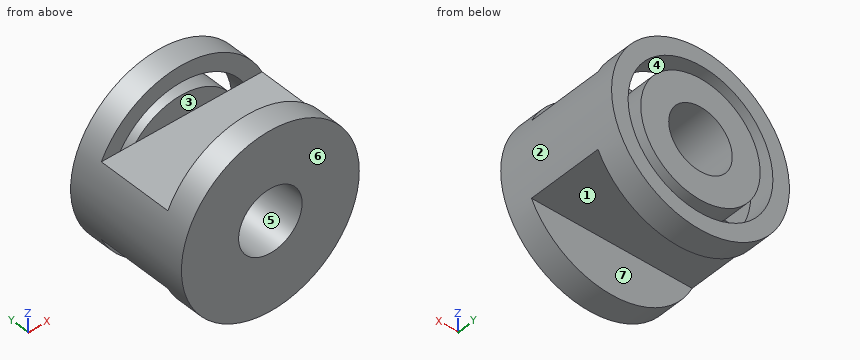
from build123d import *

# Parameters (mm, degrees)
ESQUISSE1_R                  = 3.5
BOSS_EXTRU_1_DEPTH           = 5
ESQUISSE2_R                  = 2.85
ESQUISSE2_R_2                = 2.35
ENL_V_MAT_EXTRU_1_DEPTH      = 1
ESQUISSE3_R                  = 1.25
ENL_V_MAT_EXTRU_2_DEPTH      = 6
ESQUISSE4_W                  = 2
ESQUISSE4_H                  = 3
ENL_V_MAT_EXTRU_3_DEPTH      = 4.5
ENL_V_MAT_EXTRU_3_DEPTH_BACK = 4.5


with BuildPart() as part:
    # Esquisse1 → Boss.-Extru.1 (new body)
    with BuildSketch(Plane(origin=(0, 0, 0), x_dir=(1, 0, 0), z_dir=(0, 1, 0))):
        Circle(ESQUISSE1_R)
    extrude(amount=BOSS_EXTRU_1_DEPTH)

    # Esquisse2 → Enlèv. mat.-Extru.1 (cut)
    with BuildSketch(Plane(origin=(0, 5, 0), x_dir=(1, 0, 0), z_dir=(0, 1, 0))):
        Circle(ESQUISSE2_R)
        Circle(ESQUISSE2_R_2, mode=Mode.SUBTRACT)
    extrude(amount=-ENL_V_MAT_EXTRU_1_DEPTH, mode=Mode.SUBTRACT)

    # Esquisse3 → Enlèv. mat.-Extru.2 (cut, through all)
    with BuildSketch(Plane(origin=(0, 5, 0), x_dir=(1, 0, 0), z_dir=(0, 1, 0))):
        Circle(ESQUISSE3_R)
    extrude(amount=-ENL_V_MAT_EXTRU_2_DEPTH, mode=Mode.SUBTRACT)

    # Esquisse4 → Enlèv. mat.-Extru.3 (cut, two sides)
    with BuildSketch(Plane(origin=(0, 0, 0), x_dir=(0, 0, -1), z_dir=(1, 0, 0))) as enl_v_mat_extru_3_sk:
        with Locations((-2.5, 2.5)):
            Rectangle(ESQUISSE4_W, ESQUISSE4_H)
        with Locations((2.5, 2.5)):
            Rectangle(ESQUISSE4_W, ESQUISSE4_H)
    extrude(amount=ENL_V_MAT_EXTRU_3_DEPTH, mode=Mode.SUBTRACT)
    extrude(enl_v_mat_extru_3_sk.sketch, amount=-ENL_V_MAT_EXTRU_3_DEPTH_BACK, mode=Mode.SUBTRACT)


solid = part.part
CAD build for the part. Positions are in the model's coordinates, mm. Face numbers are marked on the shaded views. A direction names the side the tool comes from. Round coordinates to 2 decimals unless told otherwise and drop trailing zeros. Loops run counter-clockwise (first coordinate to the right, second up) from the corner with the lowest first, then second, coordinate; pieces in that order, holes last. Notation, with made-up numbers: (-40, -22) - (6, -22) arc R11 ccw to (6, -12) - close; hole circle Ø3 at (6, 37). An arc over 180 degrees is marked (long way). Put each result on its own line as item: value.
1. 3-axis set-ups, long thin cutter, end or side, ignore diameter. For the marked faces 1, 2, 3 and 4: which of +Z, -Z, +X, -X, +Y, -Y reach the whole face in a straight line?
Geometry check:
face 1: -Z, +X, -X
face 2: +Y, -Y
face 3: +Z, +X, -X
face 4: +Y
2. Wall check: line 1 (X direction, y = 4.85, z = 0); line 2 (X direction, y = 1.9, z = 0). Give the ranges that are in metal, low to high.
Geometry check:
line 1: -3.5 to -2.85, -2.35 to -1.25, 1.25 to 2.35, 2.85 to 3.5
line 2: -3.5 to -1.25, 1.25 to 3.5
3. Pin check, flat tips, straight feed: P1, Ø2, axis at x = 0, z = 0, coming from the +Y side; P2, Ø1.5, axis at x = 0.5, y = 2, coming from the -Z side. Stop position of each tip, or through.
Geometry check:
P1: through
P2: z = -1.5
4. Slice it at B-B on z = 0. List the corners of the cut face in (x, y).
Geometry check:
outline: (-3.5, 0) - (-1.25, 0) - (-1.25, 5) - (-2.35, 5) - (-2.35, 4) - (-2.85, 4) - (-2.85, 5) - (-3.5, 5) - close; (1.25, 0) - (3.5, 0) - (3.5, 5) - (2.85, 5) - (2.85, 4) - (2.35, 4) - (2.35, 5) - (1.25, 5) - close
5. Slice it at A-A on x = 0. List the corners of the cut face in (y, z), and give its area (3 significant figures).
Geometry check:
outline: (0, -3.5) - (1, -3.5) - (1, -1.5) - (4, -1.5) - (4, -2.35) - (5, -2.35) - (5, -1.25) - (0, -1.25) - close; (0, 1.25) - (5, 1.25) - (5, 2.35) - (4, 2.35) - (4, 1.5) - (1, 1.5) - (1, 3.5) - (0, 3.5) - close; (4, -3.5) - (5, -3.5) - (5, -2.85) - (4, -2.85) - close; (4, 2.85) - (5, 2.85) - (5, 3.5) - (4, 3.5) - close
area: 9.50 mm²
6. Slice it at C-C on z = -2.5. List the corners of the cut face in (x, y).
Geometry check:
outline: (-2.45, 0) - (2.45, 0) - (2.45, 1) - (-2.45, 1) - close; (-2.45, 4) - (-1.37, 4) - (-1.37, 5) - (-2.45, 5) - close; (1.37, 4) - (2.45, 4) - (2.45, 5) - (1.37, 5) - close
7. Slice it at D-D on y = 1.6. List the corners of the cut face in (x, z).
Geometry check:
outline: (-3.16, -1.5) - (3.16, -1.5) arc R3.5 ccw to (3.16, 1.5) - (-3.16, 1.5) arc R3.5 ccw to start; hole circle Ø2.5 at (0, 0)
8. Two-plate mould, pull along Y, no slides. Class the marked faces 5, 6 and 7: released by +Y, released by -Y, zero draft, split by the parting line, or undercut.
Geometry check:
face 5: zero draft
face 6: released by -Y
face 7: undercut
